The drawing under review shows one solid part. Ordinate dimensions are in mm from its lowest x, y, z. A direction names the side the tool comes from. Give positions to 0.01 mm unless a question says otherwise; leave off trailing zeros. Order: outer loops, then holes, each group sorted by start corner. A loop starts at its lowest first (then second) coordinate and runs counter-clockwise, first axis right, second up. Notation, with made-up numbers: (-22.5, 61.25) -> (-8.5, 61.25) arc R37 ccw to (-8.5, 97.25) -> close; hole circle Ø10 at (88, 64). An arc over 180 degrees is marked (long way). One line per item, written item: value. Start each with the question number.
1) The part is to be moulded in two halves that separate along X. For the marked faces 6, 7 and 8, say which applies: released by +X, released by -X, zero draft, split by the parting line, or undercut.
2) Consider section A-A (x = 63). State the section outline as (y, z) points.
3) For pin 1 (2 mm diameter, centred on x = 33.5, z = 5.5, fed in from +Y) (1 decimal); pin 2 (4.5 mm diameter, centred on y = 15, z = 5, fed in from +X); pin 3 (13 mm diameter, centred on x = 56.65, y = 45.21, fed in from +Z), all flat-tipped, find the tip position at first contact; note any pin that passes through.
4) Wall thickness on line 1 along Y through (x, z) = (56, 6) (1 decimal); line 2 along X through (y, z) = (88, 3.5) (1 decimal); line 3 along X through (y, z) = (21, 2.75): over which ranges is each line inside the solid? List them lowest first. Write a range as from..to.
5) Consider section B-B (y = 42). State the section outline as (x, z) points.
6) Consider section D-D (y = 6.5). State the section outline as (x, z) points, plus the area to 3 significant figures.
7) Consider section C-C (z = 7). State the section outline as (x, y) points.
8) Tool access review of the marked faces 1, 2, 3, 4 and 5: name each direction out of +Z, -Z, +X, -X, +Y, -Y from which nothing blocks a thin tool from reaching the whole face with its end or side.
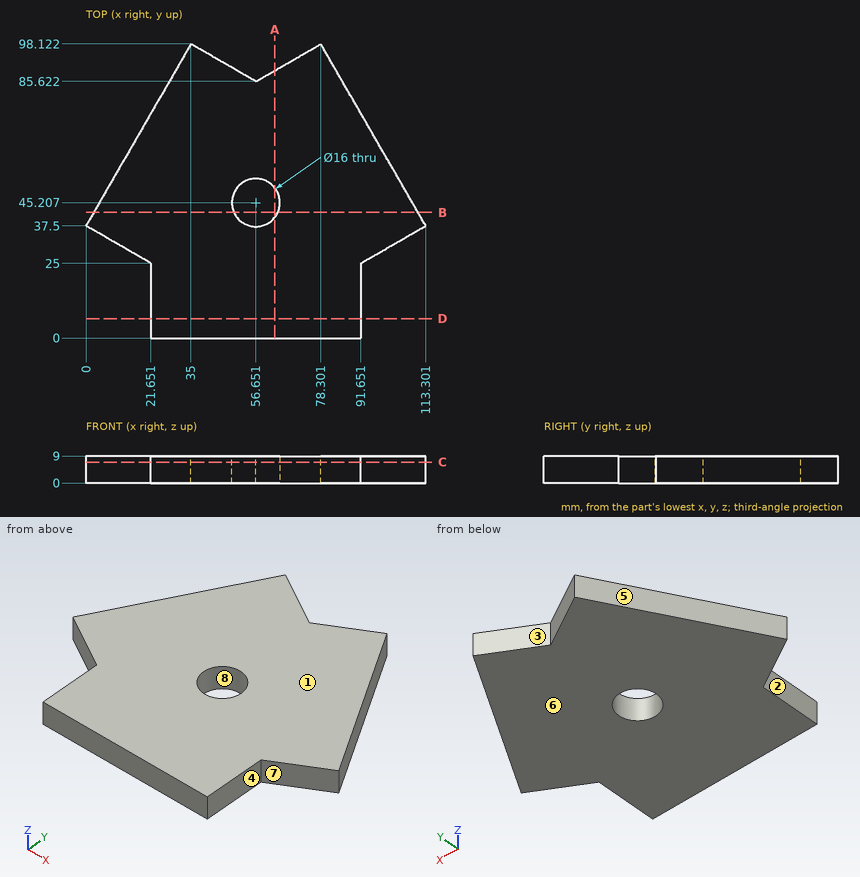
Checked values:
1. face 6: zero draft
1. face 7: released by +X
1. face 8: undercut
2. outline: (0, 0) -> (40.34, 0) -> (40.34, 9) -> (0, 9) -> close; (50.07, 0) -> (89.29, 0) -> (89.29, 9) -> (50.07, 9) -> close
3. pin 1: stops at y = 97.3
3. pin 2: stops at x = 91.65
3. pin 3: passes through
4. line 1: y = 0..37.2, 53.2..86
4. line 2: x = 29.2..52.5, 60.8..84.1
4. line 3: x = 21.65..91.65
5. outline: (2.6, 0) -> (49.32, 0) -> (49.32, 9) -> (2.6, 9) -> close; (63.98, 0) -> (110.7, 0) -> (110.7, 9) -> (63.98, 9) -> close
6. outline: (21.65, 0) -> (91.65, 0) -> (91.65, 9) -> (21.65, 9) -> close
6. area: 630 mm^2
7. outline: (0, 37.5) -> (21.65, 25) -> (21.65, 0) -> (91.65, 0) -> (91.65, 25) -> (113.3, 37.5) -> (78.3, 98.12) -> (56.65, 85.62) -> (35, 98.12) -> close; hole circle Ø16 at (56.65, 45.21)
8. face 1: +Z, +X, -X, +Y, -Y
8. face 2: +Z, -Z, -X, -Y
8. face 3: +Z, -Z, +Y
8. face 4: +Z, -Z, +X, -Y
8. face 5: +Z, -Z, -X, +Y
